```python
from build123d import *

# Parameters (mm, degrees)
F0_W     = 1351.28
F0_H     = 980.44
F1_DEPTH = 320.04
F2_R     = 12.7
F2_R_2   = 13.639748
F3_DEPTH = 467.36
F5_DEPTH = 1351.28
F6_W     = 58.42
F6_H     = 114.732094
F7_DEPTH = 1356.36


with BuildPart() as f1:
    # F0 (on Top) → F1 (new body)
    with BuildSketch(Plane.XY):
        with Locations((-251.378548, 490.22)):
            Rectangle(F0_W, F0_H)
    extrude(amount=F1_DEPTH)

    # F2 (on face) → F3 (join)
    with BuildSketch(Plane.XY.offset(320.04)):
        with Locations((94.061452, 650.24)):
            Circle(F2_R)
        with Locations((94.061452, 330.2)):
            Circle(F2_R_2)
    extrude(amount=F3_DEPTH)

    # F4 (on face) → F5 (cut)
    with BuildSketch(Plane.YZ.offset(424.261452)):
        Polygon((807.72, 254), (490.22, 254), (172.72, 254), (172.72, 0), (490.22, 0), (807.72, 0), align=None)
    extrude(amount=-F5_DEPTH, mode=Mode.SUBTRACT)

    # F6 (on face) → F7 (cut)
    with BuildSketch(Plane.YZ.offset(424.261452)):
        with Locations((29.21, 57.366047)):
            Rectangle(F6_W, F6_H)
        with Locations((951.23, 57.366047)):
            Rectangle(F6_W, F6_H)
    extrude(amount=-F7_DEPTH, mode=Mode.SUBTRACT)


solid = f1.part
```
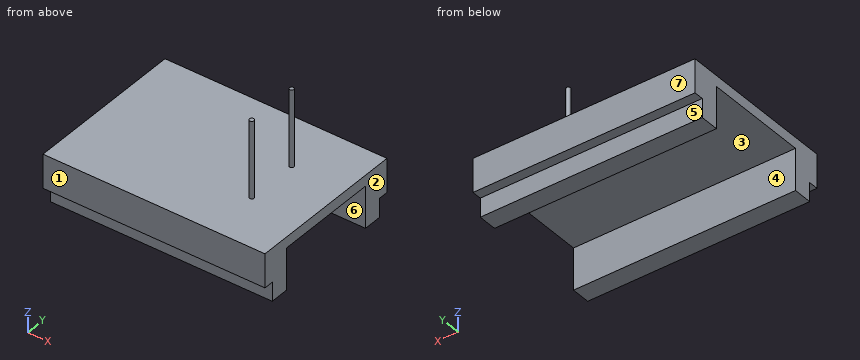
Can you work these out from the model? Positions are in its coordinate system, mm. Face numbers are marked on the shaded views. A direction names the side the tool comes from. Give positions to 0.01 mm unless a question says otherwise; leave off trailing zeros. Order: outer loops, then holes, each group sorted by start corner. A loop starts at its lowest first (then second) coordinate and runs counter-clockwise, first axis right, second up. Notation, with made-up numbers: M -26.5,-2.75 L 17.5,-2.75 A17 cw 17.5,21.25 Z; hole C 5.5,74 d2. An arc over 180 degrees is marked long. One line per item, written item: value.
1) For P1, Ø2, axis at x = -187, z = 80.5, coming from the -Y side; P2, Ø17.5, axis at x = -310.5, y = 944, coming from the -Z side, each with a flat end and sliding along its axis, tell me the tip position at first contact or that it passes through.
Answer sheet:
P1: stops at y = 58.42
P2: stops at z = 114.73
2) On a 3-axis mill with a long thin cutter (end or side, diameter ignored), from which of +Z, -Z, +X, -X, +Y, -Y can I reach the whole of each face in a straight line? I mean the marked faces 5, 6 and 7. Say none if no direction works.
Answer sheet:
face 5: -Z, +X, -X, +Y
face 6: -Z, +X, -X
face 7: +Z, -Z, +X, -X, +Y
3) I want a section at D-D, the plane y = 895.5. List the corners of the cut face in (x, z) for me, plus the area to 3 significant figures.
Answer sheet:
outline: M -927.02,0 L 424.26,0 L 424.26,320.04 L -927.02,320.04 Z
area: 432,000 mm^2
4) I want a section at C-C, the plane x = -272. List the corners of the cut face in (y, z) for me.
Answer sheet:
outline: M 0,114.73 L 58.42,114.73 L 58.42,0 L 172.72,0 L 172.72,254 L 807.72,254 L 807.72,0 L 922.02,0 L 922.02,114.73 L 980.44,114.73 L 980.44,320.04 L 0,320.04 Z
5) Please list where these lines run through material, in increasing order: line 1 along Y through (x, z) = (-868, 149.5); line 2 along Y through (x, z) = (195.5, 61); line 3 along X through (y, z) = (330, 625.5).
Answer sheet:
line 1: y = 0 to 172.72, 807.72 to 980.44
line 2: y = 58.42 to 172.72, 807.72 to 922.02
line 3: x = 80.42 to 107.7
6) I want a section at B-B, the plane z = 68.5. List the corners of the cut face in (x, y) for me, plus the area to 3 significant figures.
Answer sheet:
outline: M -927.02,58.42 L 424.26,58.42 L 424.26,172.72 L -927.02,172.72 Z; M -927.02,807.72 L 424.26,807.72 L 424.26,922.02 L -927.02,922.02 Z
area: 309,000 mm^2
7) I want a section at A-A, the plane z = 236. List the corners of the cut face in (x, y) for me, plus the area to 3 significant figures.
Answer sheet:
outline: M -927.02,0 L 424.26,0 L 424.26,172.72 L -927.02,172.72 Z; M -927.02,807.72 L 424.26,807.72 L 424.26,980.44 L -927.02,980.44 Z
area: 467,000 mm^2
8) We'd pull the mould along Y, two halves only. Please class the marked faces 1, 2, 3 and 4: released by +Y, released by -Y, zero draft, split by the parting line, or undercut.
Answer sheet:
face 1: released by -Y
face 2: zero draft
face 3: undercut
face 4: undercut
